Can you work these out from the model? Positions are in its coordinate system, mm. A direction names the side the tool comes from. Give positions to 0.01 mm unless a question says otherwise; leave off trailing zeros. Loops run counter-clockwise (first coordinate to the right, second up) from the corner with the lowest first, then second, coordinate; pieces in that order, holes last. Notation, with made-up numbers: (58.5, 43.5) - (73.5, 43.5) arc R29 ccw to (73.5, 67.5) - close; hole circle Ø9 at (85, 19.25). An arc over 180 degrees is marked (long way). Use a Markdown table: item, result. Add a question column.
```python
from build123d import *

# Parameters (mm, degrees)
BOSS_EXTRUDE1_DEPTH        = 1
CUT_EXTRUDE1_REACH         = 3
SKETCH2_R                  = 1.65
CHAMFER1_SIZE              = 0.3
F_1_2_1_2_DIAMETER_HOLE1_D = 1.2


with BuildPart() as part:
    # Sketch1 → Boss-Extrude1 (new body)
    with BuildSketch(Plane.XY):
        with BuildLine():
            Line((0, 3), (-4.635898385, 3))
            ThreePointArc((-4.635898385, 3), (-6.135898385, 2.598076211), (-7.233974596, 1.5))
            Line((-7.233974596, 1.5), (-8.1, 0))
            Line((-8.1, 0), (-6.665673326, 0.384326674))
            Line((-6.665673326, 0.384326674), (-1.5, -2.598076211))
            ThreePointArc((-1.5, -2.598076211), (2.897777479, -0.776457135), (0, 3))
        make_face()
    extrude(amount=-BOSS_EXTRUDE1_DEPTH)

    # Sketch2 → Cut-Extrude1 (cut, up to next)
    with BuildSketch(Plane.XY, mode=Mode.PRIVATE) as cut_extrude1_sk1:
        Circle(SKETCH2_R)
    cut_extrude1_tool1 = extrude(cut_extrude1_sk1.sketch, amount=-CUT_EXTRUDE1_REACH, mode=Mode.PRIVATE) & part.part
    add(cut_extrude1_tool1.solids().sort_by_distance((0, 0, 0))[0], mode=Mode.SUBTRACT)

    # Chamfer1
    chamfer1_edges = [part.edges().sort_by_distance(p)[0] for p in [
        (-1.65, 0, 0),
    ]]
    chamfer(chamfer1_edges, length=CHAMFER1_SIZE)

    # Ø1.2 (1.2) Diameter Hole1 (through all)
    with Locations(Plane.XY):
        with Locations((-2.801184896, 0.750575231)):
            Hole(F_1_2_1_2_DIAMETER_HOLE1_D / 2)


solid = part.part
```
1. Will this pin go through, and if not, where does the flat tip stop? P1, Ø3, axis at x = 0, y = 0, coming from the +Z side.
2. Suppose I cut it at B-B (y = 1.2). State how many separate pieces and enclosed holes the cut face has, and give its area (3 significant figures).
3. Suppose I cut it at A-A (z = -0.65). List the corners of the cut face in (x, y) for me, and give its area (3 significant figures).
4. Suppose I cut it at D-D (x = -7.5). List the corners of the cut face in (y, z) for me, and give its area (3 significant figures).
5. Please list where these lines run through material, in increasing order: line 1 along X through (y, z) = (0.5, -0.55); line 2 along X through (y, z) = (0.95, -0.5); line 3 along Y through (x, z) = (-1.5, -0.45). Write a range as [from, to].
6. Suppose I cut it at C-C (z = -0.15). List the corners of the cut face in (x, y) for me, and give its area (3 significant figures).
7. If we mould it in two halves opening along Y, with no side actions, what happens to faces 1 (the face through (-1.216, 1.115, -0.645)), 2 (the face through (-3, 0, 0)), 3 (the face through (2.877, -0.851, -0.493))? For each: released by +Y, released by -Y, zero draft, split by the parting line, or undercut.
8. On a 3-axis mill with a long thin cutter (end or side, diameter ignored), from which of +Z, -Z, +X, -X, +Y, -Y can I reach the whole of each face in a straight line? I mean faces 4 (the face through (-7.39, 0.19, -0.49)), 5 (the face through (-7.66, 0.76, -0.49)). Say none if no direction works.
Results below:
| question | item | result |
|---|---|---|
| 1 | P1 | through |
| 2 | separate pieces | 3 |
| 2 | enclosed holes | 0 |
| 2 | area | 6.97 mm² |
| 3 | outline | (-8.1, 0) - (-6.67, 0.38) - (-1.5, -2.6) arc R3 ccw (long way) to (0, 3) - (-4.64, 3) arc R3 ccw to (-7.23, 1.5) - close; hole circle Ø1.2 at (-2.8, 0.75); hole circle Ø3.3 at (0, 0) |
| 3 | area | 35.4 mm² |
| 4 | outline | (0.16, -1) - (1.04, -1) - (1.04, 0) - (0.16, 0) - close |
| 4 | area | 0.878 mm² |
| 5 | line 1 | [-7.81, -3.35], [-2.26, -1.57], [1.57, 2.96] |
| 5 | line 2 | [-7.55, -3.37], [-2.24, -1.35], [1.35, 2.85] |
| 5 | line 3 | [-2.6, -0.69], [0.69, 3] |
| 6 | outline | (-8.1, 0) - (-6.67, 0.38) - (-1.5, -2.6) arc R3 ccw (long way) to (0, 3) - (-4.64, 3) arc R3 ccw to (-7.23, 1.5) - close; hole circle Ø1.2 at (-2.8, 0.75); hole circle Ø3.6 at (0, 0) |
| 6 | area | 33.8 mm² |
| 7 | face 1 | undercut |
| 7 | face 2 | zero draft |
| 7 | face 3 | split by the parting line |
| 8 | face 4 | +Z, -Z, -Y |
| 8 | face 5 | +Z, -Z, -X, +Y |
